For this review, take the finished solid that the model builds, in its own axes (mm). Face numbers are marked on the shaded views. A direction names the side the tool comes from. Coordinates: 2 decimals unless noted, no trailing zeros. Loops run counter-clockwise (first coordinate to the right, second up) from the corner with the lowest first, then second, coordinate; pieces in that order, holes last. Notation, with made-up numbers: M -17.5,21 L 21.5,21 A26 cw 21.5,50 Z; hole C -32,58.25 d2. An arc over 180 degrees is marked long. Write item = value, one per line.
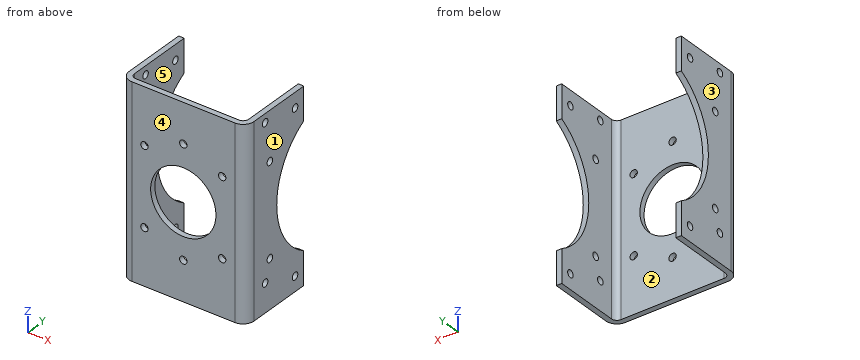
Autodesk Inventor part; units mm, degrees
ref_plane "YZ Plane" through (0, 0, 0) normal (1, 0, 0) x (0, 1, 0)
ref_plane "XZ Plane" through (0, 0, 0) normal (0, 1, 0) x (-1, 0, 0)
ref_plane "XY Plane" through (0, 0, 0) normal (0, 0, 1) x (1, 0, 0)
sketch "スケッチ1" plane through (0, 0, 0) normal (0, 1, 0) x (-1, 0, 0)
  line L0 (30, 55) -> (-30, 55)
  line L1 (-30, 55) -> (-30, -55)
  line L2 (-30, -55) -> (30, -55)
  line L3 (30, -55) -> (30, 55)
  line L4 (30, 55) -> (-30, -55) construction
  line L5 (-30, 55) -> (30, -55) construction
  point P0 (0, 0)
  dimension "d0" = 60
  dimension "d1" = 110
extrude "プレート1" add sketch "スケッチ1" along normal blind 3.2
sketch "スケッチ2" plane through (-33.2, 6.4, 55) normal (-1, 0, 0) x (0, -1, 0)
  line L0 (0, -110) -> (0, 0)
  line L1 (0, 0) -> (-193.6, 0)
  line L2 (-193.6, 0) -> (-193.6, -110)
  line L3 (-193.6, -110) -> (0, -110)
edge flange "フランジ1" height 200 angle 90 thickness 3.2 bend radius 3.2 thickness toward (-1, 0, 0) relief tear relief width 3.2 relief depth 1.6 corner gap 3.2 corner form 0 edges at (-30, 3.2, 0) (30, 3.2, 0) wall of the first edge with corners at (-33.2, 6.4, -55) (-33.2, 6.4, 55) (-33.2, 200, 55) (-33.2, 200, -55)
bend "曲げ1"
corner "コーナー1"
sketch "スケッチ3" plane through (36.4, 200, 55) normal (1, 0, 0) x (0, 0, -1)
  circle A0 centre (55, -135) radius 41
  line L0 (0, -200) -> (110, -200)
  line L1 (0, -193.6) -> (0, 0)
  line L2 (110, 0) -> (110, -193.6)
  line L3 (0, 0) -> (0, -193.6)
  line L4 (110, 0) -> (0, 0)
  line L5 (0, -155) -> (110, -155)
  line L6 (110, -155) -> (110, 0)
  line L7 (110, 0) -> (0, 0)
  line L8 (0, 0) -> (0, -155)
  point P0 (55, -200)
  point P1 (90.7911, -155)
  point P2 (110, -155)
  point P3 (0, -155)
  point P4 (19.2089, -155)
  dimension "d13" = 82
  dimension "d14" = 65
  dimension "d17" = 45
extrude "押し出し1" cut sketch "スケッチ3" against normal through all
sketch "スケッチ4" plane through (36.4, 6.4, 55) normal (1, 0, 0) x (0, 0, -1)
  arc A0 (19.2089, 38.6) -> (90.7911, 38.6) centre (55, 58.6) ccw
  circle A1 centre (55, 58.6) radius 53.5
  point P0 (55, -6.4)
  point P1 (55, 112.1)
  point P2 (28.25, 104.9324)
  point P3 (8.6676, 85.35)
  point P4 (1.5, 58.6)
  point P5 (8.6676, 31.85)
  point P6 (28.25, 12.2676)
  point P7 (55, 5.1)
  point P8 (81.75, 12.2676)
  point P9 (101.3324, 31.85)
  point P10 (108.5, 58.6)
  point P11 (101.3324, 85.35)
  point P12 (81.75, 104.9324)
  dimension "d18" = 107
  dimension "d21" = 360
hole "穴1" at (36.4, 18.6676, 26.75) at (36.4, 38.25, 46.3324) at (36.4, 38.25, -46.3324) at (36.4, 18.6676, -26.75) direction (-1, 0, 0) diameter 4.3 end through all
sketch "スケッチ5" plane through (36.4, 6.4, 55) normal (1, 0, 0) x (0, 0, -1)
  line L0 (0, 0) -> (0, 38.6)
  arc A0 (19.2089, 38.6) -> (90.7911, 38.6) centre (55, 58.6) ccw
  line L1 (0, 0) -> (110, 0)
  point P0 (55, -6.4)
  point P1 (5, 8.6)
  point P2 (93.4, 8.6)
  dimension "d30" = 88.4
  dimension "d31" = 5
  dimension "d34" = 50
hole "穴2" at (36.4, 15, 50) at (36.4, 15, -38.4) direction (-1, 0, 0) diameter 4.3 end through all
sketch "スケッチ6" plane through (0, 0, 0) normal (0, -1, 0) x (1, 0, 0)
  circle A0 centre (0, 0) radius 32
  point P0 (0, 32)
  point P1 (-22.6274, 22.6274)
  point P2 (-32, 0)
  point P3 (-22.6274, -22.6274)
  point P4 (0, -32)
  point P5 (22.6274, -22.6274)
  point P6 (32, 0)
  point P7 (22.6274, 22.6274)
  dimension "d42" = 64
  dimension "d45" = 360
hole "穴3" at (22.6274, 0, 22.6274) at (-22.6274, 0, 22.6274) at (0, 0, 32) at (22.6274, 0, -22.6274) at (0, 0, -32) at (-22.6274, 0, -22.6274) direction (0, 1, 0) diameter 4.3 end through all
sketch "スケッチ7" plane through (0, 3.2, 0) normal (0, 1, 0) x (1, 0, 0)
  circle A0 centre (0, 0) radius 19
  dimension "d54" = 38
extrude "押し出し2" cut sketch "スケッチ7" against normal blind 10
equation "\"d28\" = Thickness"
equation "\"d2\" = Thickness"
equation "\"d3\" = BendReliefWidth"
equation "\"d4\" = BendReliefDepth"
equation "\"d5\" = MinimumRemnant"
equation "\"d6\" = TransitionRadius"
equation "\"d9\" = BendRadius"
equation "\"d10\" = CornerReliefSize"
equation "\"d11\" = GapSize"
equation "\"d12\" = JacobiRadiusSize"
equation "\"BendRadius\" = Thickness"
equation "\"BendReliefWidth\" = Thickness"
equation "\"BendReliefDepth\" = 0.5 * Thickness"
equation "\"CornerReliefSize\" = 4 * Thickness"
equation "\"MinimumRemnant\" = 2 * Thickness"
equation "\"TransitionRadius\" = BendRadius"
equation "\"JacobiRadiusSize\" = BendRadius"
equation "\"GapSize\" = Thickness"
properties part number "steelplate2" material "鋼、炭素鋼"
Q1. Draft analysis for pull direction X (two halves, no side actions). For the marked faces 3, 4 and 5, state which applies: +X half, -X half, draft (parallel to the pull), parting line (faces both ways), or undercut.
Solved:
face_3 = -X half
face_4 = draft
face_5 = undercut
Q2. For line 1 along Z through (x, y) = (35.2, 15); line 2 along Z through (x, y) = (0, 0.95); line 3 along X through (y, z) = (18.5, 39.5), list the stretches that pass through material, from the lowest coordinate up.
Solved:
line_1 = -55 to -40.55, -36.25 to 47.85, 52.15 to 55
line_2 = -55 to -34.15, -29.85 to -19, 19 to 29.85, 34.15 to 55
line_3 = -36.4 to -33.2, 33.2 to 36.4
Q3. For pin 1 Ø4 at (y, z) = (15, 50) entering from -X; pin 2 Ø5 at (y, z) = (38.25, 46.33) entering from -X; pin 3 Ø2 at (x, z) = (11.5, -21) entering from +Y, all flat-tipped, find the tip position at first contact; note any pin that passes through.
Solved:
pin_1 = through
pin_2 = -36.4
pin_3 = 3.2
Q4. Add section A-A (y = 15). Write out the cut boundary in (x, z).
Solved:
outline = M -36.4,-55 L -33.2,-55 L -33.2,-40.55 L -36.4,-40.55 Z; M -36.4,-36.25 L -33.2,-36.25 L -33.2,47.85 L -36.4,47.85 Z; M -36.4,52.15 L -33.2,52.15 L -33.2,55 L -36.4,55 Z; M 33.2,-55 L 36.4,-55 L 36.4,-40.55 L 33.2,-40.55 Z; M 33.2,-36.25 L 36.4,-36.25 L 36.4,47.85 L 33.2,47.85 Z; M 33.2,52.15 L 36.4,52.15 L 36.4,55 L 33.2,55 Z
Q5. Add section D-D (x = 9.5). Write out the cut boundary in (y, z).
Solved:
outline = M 0,-55 L 3.2,-55 L 3.2,-16.45 L 0,-16.45 Z; M 0,16.45 L 3.2,16.45 L 3.2,55 L 0,55 Z
Q6. Add section C-C (z = 50). Write out the cut boundary in (x, y), and give its area (3 significant figures).
Solved:
outline = M -36.4,6.4 A6.4 ccw -30,0 L 30,0 A6.4 ccw 36.4,6.4 L 36.4,12.85 L 33.2,12.85 L 33.2,6.4 A3.2 cw 30,3.2 L -30,3.2 A3.2 cw -33.2,6.4 L -33.2,12.85 L -36.4,12.85 Z; M -36.4,17.15 L -33.2,17.15 L -33.2,45 L -36.4,45 Z; M 33.2,17.15 L 36.4,17.15 L 36.4,45 L 33.2,45 Z
area = 460 mm²
Q7. Add section B-B (x = 0). Write out the cut boundary in (y, z).
Solved:
outline = M 0,-55 L 3.2,-55 L 3.2,-34.15 L 0,-34.15 Z; M 0,-29.85 L 3.2,-29.85 L 3.2,-19 L 0,-19 Z; M 0,19 L 3.2,19 L 3.2,29.85 L 0,29.85 Z; M 0,34.15 L 3.2,34.15 L 3.2,55 L 0,55 Z
Q8. Machinability: for the marked faces 1 and 2, which of the approach directions +Z, -Z, +X, -X, +Y, -Y give a long, thin tool a straight path to every point of the face, cutting with its end or side? Answer none if there is none.
Solved:
face_1 = +Z, -Z, +X, +Y, -Y
face_2 = +Z, -Z, +Y
